```python
from build123d import *

# Parameters (mm, degrees)
F0_W     = 50.8
F0_H     = 69.85
F1_DEPTH = 19.05
F2_R     = 5.08
F3_R     = 5.08


with BuildPart() as f1:
    # F0 (on Front) → F1 (new body)
    with BuildSketch(Plane.XZ):
        with Locations((-25.4, 34.925)):
            Rectangle(F0_W, F0_H)
    extrude(amount=F1_DEPTH)

    # F2
    f2_edges = [f1.edges().sort_by_distance(p)[0] for p in [
        (0, -9.525, 69.85),
        (-50.8, -9.525, 69.85),
        (-25.4, 0, 69.85),
        (-25.4, -19.05, 69.85),
    ]]
    fillet(f2_edges, radius=F2_R)

    # F3
    f3_edges = [f1.edges().sort_by_distance(p)[0] for p in [
        (-50.8, -9.525, 0),
        (0, -9.525, 0),
        (-25.4, 0, 0),
        (-25.4, -19.05, 0),
    ]]
    fillet(f3_edges, radius=F3_R)


solid = f1.part
```
Input: part model. Units: mm. Frame: model coordinates. Round coordinates to 2 decimals unless told otherwise and drop trailing zeros. Loops run counter-clockwise (first coordinate to the right, second up) from the corner with the lowest first, then second, coordinate; pieces in that order, holes last. Notation, with made-up numbers: M 4,54 L 47,54 A24 cw 47,85 Z; hole C 36,73 d11. An arc over 180 degrees is marked long. Answer in a Markdown table with one row per item. Add a question column.
1. Ray query, probe 1 along Z at (x, y) = (-33, -3.75); probe 2 along X at (y, z) = (-18, 66); probe 3 along Y at (x, z) = (-20, 66.5). Return the intervals inside material, ascending.
2. Section B-B (y = -3). Output: boundary loops of the cut face in (x, z).
3. Section A-A (x = -29.5). Output: boundary loops of the cut face in (y, z).
Values follow:
| question | item | result |
|---|---|---|
| 1 | probe 1 | 0.18 to 69.67 |
| 1 | probe 2 | -50.65 to -0.15 |
| 1 | probe 3 | -18.75 to -0.3 |
| 2 | outline | M -50.8,5.08 A5.08 ccw -47.8,0.45 L -3,0.45 A5.08 ccw 0,5.08 L 0,64.77 A5.08 ccw -3,69.4 L -47.8,69.4 A5.08 ccw -50.8,64.77 Z |
| 3 | outline | M -19.05,5.08 A5.08 ccw -13.97,0 L -5.08,0 A5.08 ccw 0,5.08 L 0,64.77 A5.08 ccw -5.08,69.85 L -13.97,69.85 A5.08 ccw -19.05,64.77 Z |
